Source: CAD feature listing. Evaluate the final solid. Frame: model axes, mm. A direction names the side the tool comes from. Give positions to 0.01 mm unless a question says otherwise; leave off trailing zeros. Write each loop counter-clockwise with the first axis right and the second up, starting at its lowest first coordinate (ties: lowest second). Pieces come first, ordered by that corner, then holes. Notation, with made-up numbers: M 54.25,86 L 69.25,86 A26 cw 69.25,112 Z; hole C 19,0 d6. An arc over 180 degrees is marked long. Return JSON: item names as keys, results as strings.
```python
from build123d import *

# Parameters (mm, degrees)
F0_R     = 3.175
F0_R_2   = 1.5875
F1_DEPTH = 3.048


with BuildPart() as f1:
    # F0 (on Front) → F1 (new body)
    with BuildSketch(Plane.XZ):
        with BuildLine():
            ThreePointArc((-9.450293, 115.490625), (-0.596483, 104.793695), (9.525, 114.3))
            ThreePointArc((9.525, 114.3), (9.506305, 114.896483), (9.450293, 115.490625))
            ThreePointArc((9.450293, 115.490625), (0, 123.825), (-9.450293, 115.490625))
        make_face()
        with Locations((0, 114.3)):
            Circle(F0_R, mode=Mode.SUBTRACT)
        with BuildLine():
            ThreePointArc((9.450293, 115.490625), (9.506305, 114.896483), (9.525, 114.3))
            ThreePointArc((9.525, 114.3), (-0.596483, 104.793695), (-9.450293, 115.490625))
            Line((-9.450293, 115.490625), (-15.750488, 65.484375))
            ThreePointArc((-15.750488, 65.484375), (0, 79.375), (15.750488, 65.484375))
            Line((15.750488, 65.484375), (9.450293, 115.490625))
        make_face()
        with Locations((-1.5875, 100.0252)):
            Circle(F0_R_2, mode=Mode.SUBTRACT)
        with BuildLine():
            ThreePointArc((15.875, 63.5), (15.843841, 64.494139), (15.750488, 65.484375))
            ThreePointArc((15.750488, 65.484375), (0, 79.375), (-15.750488, 65.484375))
            ThreePointArc((-15.750488, 65.484375), (-15.875, 63.5), (-15.750488, 61.515625))
            ThreePointArc((-15.750488, 61.515625), (0, 47.625), (15.750488, 61.515625))
            ThreePointArc((15.750488, 61.515625), (15.843841, 62.505861), (15.875, 63.5))
        make_face()
        with Locations((0, 63.5)):
            Circle(F0_R, mode=Mode.SUBTRACT)
        with BuildLine():
            ThreePointArc((15.750488, 61.515625), (0, 47.625), (-15.750488, 61.515625))
            Line((-15.750488, 61.515625), (-7.875244, -0.992188))
            ThreePointArc((-7.875244, -0.992188), (-0.497069, 7.921921), (7.9375, 0))
            ThreePointArc((7.9375, 0), (5.61266, -5.61266), (0, -7.9375))
            Line((0, -7.9375), (44.45, -7.9375))
            ThreePointArc((44.45, -7.9375), (36.5125, 0), (44.45, 7.9375))
            Line((44.45, 7.9375), (18.014958, 7.9375))
            ThreePointArc((18.014958, 7.9375), (12.052308, 10.629137), (10.127114, 16.881475))
            Line((10.127114, 16.881475), (15.750488, 61.515625))
        make_face()
        with BuildLine():
            ThreePointArc((7.9375, 0), (-0.497069, 7.921921), (-7.875244, -0.992188))
            ThreePointArc((-7.875244, -0.992188), (-5.250163, -5.953125), (0, -7.9375))
            ThreePointArc((0, -7.9375), (5.61266, -5.61266), (7.9375, 0))
        make_face()
        Circle(F0_R, mode=Mode.SUBTRACT)
        with BuildLine():
            ThreePointArc((44.45, 7.9375), (36.5125, 0), (44.45, -7.9375))
            ThreePointArc((44.45, -7.9375), (50.06266, -5.61266), (52.3875, 0))
            ThreePointArc((52.3875, 0), (50.06266, 5.61266), (44.45, 7.9375))
        make_face()
        with Locations((44.45, 0)):
            Circle(F0_R, mode=Mode.SUBTRACT)
    extrude(amount=F1_DEPTH)


solid = f1.part
```
1) Cut plane A-A, the plane z = 114.3. Return the cut outline in (x, y) (3 decimals).
Numbers:
{"outline": "M -9.6,-3.048 L -3.175,-3.048 L -3.175,0 L -9.6,0 Z; M 3.175,-3.048 L 9.6,-3.048 L 9.6,0 L 3.175,0 Z"}
2) Line query: line 1 (Z direction, x = -1, y = -1.55); line 2 (Z direction, x = 28.5, y = -0.85); line 3 (X direction, y = -0.95, z = 100). Output: solid intervals per line, ascending. Write a range as [from, to].
Numbers:
{"line 1": "z = [-7.87, -3.01], [3.01, 60.49], [66.51, 98.55], [101.5, 111.29], [117.31, 123.77]", "line 2": "z = [-7.94, 7.94]", "line 3": "x = [-11.4, -3.17], [0, 11.4]"}
3) Draft query along Z for faces 1 (the face through (0.193, -1.503, 123.823)), 2 (the face through (-1.932, -1.503, 98.475)), 3 (the face through (-5.31, -1.5, -5.9)), 4 (the face through (-0.69, -1.5, -3.1)). Return one class per face: released by +Z, released by -Z, zero draft, split by the parting line, or undercut.
Numbers:
{"face 1": "released by +Z", "face 2": "undercut", "face 3": "released by -Z", "face 4": "undercut"}
4) Cut plane D-D, the plane x = 6. Return the cut outline in (y, z).
Numbers:
{"outline": "M -3.05,-7.94 L 0,-7.94 L 0,121.7 L -3.05,121.7 Z"}
5) Contact query for flat-ended pins moving along their axis: pin 1 Ø1.5 at (x, y) = (35, -2) entering from +Z; pin 2 Ø1.5 at (y, z) = (-1, 82) entering from +X; pin 3 Ø4 at (x, z) = (0, 114.3) entering from +Y; pin 4 Ø1 at (y, z) = (-2, 15) entering from -X. Output: stop coordinate, or through.
Numbers:
{"pin 1": "stops at z = 7.94", "pin 2": "stops at x = 13.76", "pin 3": "passes through", "pin 4": "stops at x = -9.95"}
6) Cut plane C-C, the plane z = 80.5. Return the cut outline in (x, y).
Numbers:
{"outline": "M -13.86,-3.05 L 13.86,-3.05 L 13.86,0 L -13.86,0 Z"}
7) Set-up query: faces 5 (the face through (12.9, -1.5, 38.9)), 6 (the face through (3, 0, 59)), 7 (the face through (31, -2, 7.938)). Return all of +Z, -Z, +X, -X, +Y, -Y with unobstructed straight access to the full face (end or side cutting, diameter ignored); none if empty.
Numbers:
{"face 5": "+X, +Y, -Y", "face 6": "+Z, -Z, +X, -X, +Y", "face 7": "+Z, +X, +Y, -Y"}
8) Cut plane B-B, the plane y = -2.4. Give the number of separate pieces and of enclosed holes in the cut face, then the cut area to 3 significant figures.
Numbers:
{"separate pieces": "1", "enclosed holes": "5", "area": "3,640 mm²"}
